Design review of the part built by this model. Coordinates are the model's own, in mm. Round coordinates to 2 decimals unless told otherwise and drop trailing zeros. Loops run counter-clockwise (first coordinate to the right, second up) from the corner with the lowest first, then second, coordinate; pieces in that order, holes last. Notation, with made-up numbers: (-5, 59.5) - (24, 59.5) arc R15 cw to (24, 63.5) - close; hole circle Ø6 at (51, 22). An arc over 180 degrees is marked (long way). Return JSON: item names as keys, results as strings. Group by question number.
from build123d import *

# Parameters (mm, degrees)
SKETCH1_W           = 250
SKETCH1_H           = 200
BOSS_EXTRUDE1_DEPTH = 4
SKETCH4_R           = 5
CUT_EXTRUDE1_DEPTH  = 5
SKETCH9_R           = 2
CUT_EXTRUDE5_DEPTH  = 5
FILLET1_R           = 10


with BuildPart() as part:
    # Sketch1 → Boss-Extrude1 (new body)
    with BuildSketch(Plane(origin=(0, 0, 0), x_dir=(1, 0, 0), z_dir=(0, 1, 0))):
        with Locations((275, 105.323868678)):
            Rectangle(SKETCH1_W, SKETCH1_H)
    extrude(amount=BOSS_EXTRUDE1_DEPTH)

    # Sketch4 → Cut-Extrude1 (cut, through all)
    with BuildSketch(Plane(origin=(0, 4, 0), x_dir=(1, 0, 0), z_dir=(0, 1, 0))):
        with Locations((360, 37.823868678)):
            Circle(SKETCH4_R)
        with Locations((180, 37.823868678)):
            Circle(SKETCH4_R)
        with Locations((360, 172.823868678)):
            Circle(SKETCH4_R)
        with Locations((180, 172.823868678)):
            Circle(SKETCH4_R)
    extrude(amount=-CUT_EXTRUDE1_DEPTH, mode=Mode.SUBTRACT)

    # Sketch9 → Cut-Extrude5 (cut, through all)
    with BuildSketch(Plane.XZ):
        with Locations((155.1, -196.823868678)):
            Circle(SKETCH9_R)
        with Locations((155.1, -182.823868678)):
            Circle(SKETCH9_R)
        with Locations((171.1, -196.823868678)):
            Circle(SKETCH9_R)
        with Locations((171.1, -182.823868678)):
            Circle(SKETCH9_R)
        with Locations((155.1, -27.823868678)):
            Circle(SKETCH9_R)
        with Locations((155.1, -13.823868678)):
            Circle(SKETCH9_R)
        with Locations((171.1, -13.823868678)):
            Circle(SKETCH9_R)
        with Locations((171.1, -27.823868678)):
            Circle(SKETCH9_R)
        with Locations((394.9, -182.823868678)):
            Circle(SKETCH9_R)
        with Locations((394.9, -196.823868678)):
            Circle(SKETCH9_R)
        with Locations((378.9, -196.823868678)):
            Circle(SKETCH9_R)
        with Locations((378.9, -182.823868678)):
            Circle(SKETCH9_R)
        with Locations((394.9, -27.823868678)):
            Circle(SKETCH9_R)
        with Locations((378.9, -27.823868678)):
            Circle(SKETCH9_R)
        with Locations((378.9, -13.823868678)):
            Circle(SKETCH9_R)
        with Locations((394.9, -13.823868678)):
            Circle(SKETCH9_R)
    extrude(amount=-CUT_EXTRUDE5_DEPTH, mode=Mode.SUBTRACT)

    # Fillet1
    fillet1_edges = [part.edges().sort_by_distance(p)[0] for p in [
        (150, 2, -205.323868678),
        (400, 2, -205.323868678),
        (400, 2, -5.323868678),
        (150, 2, -5.323868678),
    ]]
    fillet(fillet1_edges, radius=FILLET1_R)


solid = part.part
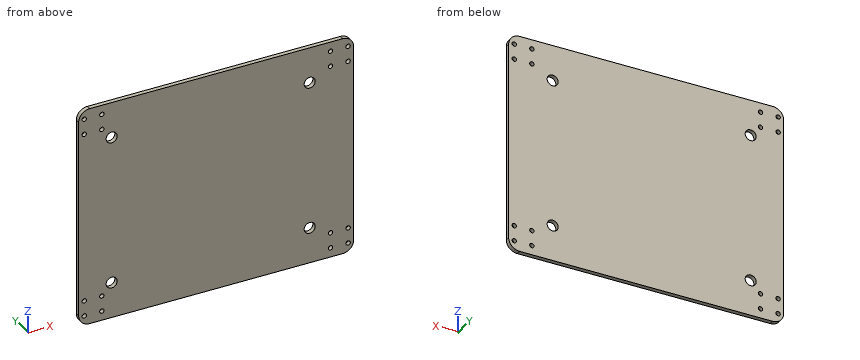
Q1. Insertion check: pin 1 Ø16 at (x, z) = (180, -172.82) entering from +Y; pin 2 Ø8 at (x, z) = (360, -37.82) entering from -Y. Each pin has a flat end and moves straight along its axis. Give the tip position at first contact, or say it passes through.
Q2. Add section A-A, the plane x = 180. State the section outline as (y, z) points.
Q3. For line 1 (Z direction, x = 378.9, y = 2); line 2 (Z direction, x = 180, y = 1.6); line 3 (Z direction, x = 155.1, y = 1.3), list the stretches that pass through material, from the lowest coordinate up.
Evaluation:
{
 "1": {"pin 1": "y = 4", "pin 2": "through"},
 "2": {"outline": "(0, -205.32) - (4, -205.32) - (4, -177.82) - (0, -177.82) - close; (0, -167.82) - (4, -167.82) - (4, -42.82) - (0, -42.82) - close; (0, -32.82) - (4, -32.82) - (4, -5.32) - (0, -5.32) - close"},
 "3": {"line 1": "-205.32 to -198.82, -194.82 to -184.82, -180.82 to -29.82, -25.82 to -15.82, -11.82 to -5.32", "line 2": "-205.32 to -177.82, -167.82 to -42.82, -32.82 to -5.32", "line 3": "-204.04 to -198.82, -194.82 to -184.82, -180.82 to -29.82, -25.82 to -15.82, -11.82 to -6.61"}
}
